```python
from build123d import *

# Parameters (mm, degrees)
SKETCH1_W           = 10
SKETCH1_H           = 10
BOSS_EXTRUDE1_DEPTH = 50
SKETCH3_R           = 4.25
BOSS_EXTRUDE2_DEPTH = 140
CHAMFER1_SIZE       = 1
SKETCH7_R           = 4
CUT_EXTRUDE3_DEPTH  = 4.5
SKETCH7_5_R         = 2.25
CUT_EXTRUDE4_DEPTH  = 20


with BuildPart() as part:
    # Sketch1 → Boss-Extrude1 (new body)
    with BuildSketch(Plane(origin=(0, 0, 0), x_dir=(0, 0, -1), z_dir=(1, 0, 0))):
        Rectangle(SKETCH1_W, SKETCH1_H)
    extrude(amount=BOSS_EXTRUDE1_DEPTH)

    # Sketch3 → Boss-Extrude2 (add)
    with BuildSketch(Plane(origin=(50, 0, 0), x_dir=(0, 0, -1), z_dir=(1, 0, 0))):
        Circle(SKETCH3_R)
    extrude(amount=BOSS_EXTRUDE2_DEPTH)

    # Chamfer1
    chamfer1_edges = [part.edges().sort_by_distance(p)[0] for p in [
        (190, 0, 4.25),
    ]]
    chamfer(chamfer1_edges, length=CHAMFER1_SIZE)

    # Sketch5 → Cut-Revolve1 (revolve, cut)
    with BuildSketch(Plane(origin=(0, 0, 0), x_dir=(-1, 0, 0), z_dir=(0, -0.7071067811865476, -0.7071067811865476))):
        Polygon((-50, 7.071067812), (-50, 6.571067812), (-49.5, 7.071067812), align=None)
    revolve(axis=Axis((-14.523088714, 0, 0), (1, 0, 0)), mode=Mode.SUBTRACT)

    # Sketch7 → Cut-Extrude3 (cut)
    with BuildSketch(Plane(origin=(0, 0, -5), x_dir=(-1, 0, 0), z_dir=(0, 0, -1))):
        with Locations(Location((-5, 0, 0), (0, 0, 90))):
            Circle(SKETCH7_R)
    extrude(amount=-CUT_EXTRUDE3_DEPTH, mode=Mode.SUBTRACT)

    # Sketch7_5 → Cut-Extrude4 (cut)
    with BuildSketch(Plane(origin=(0, 0, -5), x_dir=(-1, 0, 0), z_dir=(0, 0, -1))):
        with Locations(Location((-5, 0, 0), (0, 0, 90))):
            Circle(SKETCH7_5_R)
    extrude(amount=-CUT_EXTRUDE4_DEPTH, mode=Mode.SUBTRACT)


solid = part.part
```
CAD build for the part. Positions are in the model's coordinates, mm. A direction names the side the tool comes from. Coordinates: 2 decimals unless noted, no trailing zeros. Write each loop counter-clockwise with the first axis right and the second up, starting at its lowest first coordinate (ties: lowest second). Pieces come first, ordered by that corner, then holes. Notation, with made-up numbers: (68.5, -4.75) -> (111.5, -4.75) arc R19 ccw to (111.5, 5.25) -> close; hole circle Ø5 at (89.5, -20.5). An arc over 180 degrees is marked (long way). Use CSV: the item, a comma, the result in double quotes. Start each with the question number.
Item 1: Band-saw the part on C-C, the plane x = 96. Write the cut outline in (y, z), plus the area to 3 significant figures.
Item 2: Band-saw the part on B-B, the plane x = 5. Write the cut outline in (y, z), plus the area to 4 significant figures.
Item 3: Drop flat-ended pins along their axis: P1, Ø5, axis at x = 5, y = 0, coming from the +Z side; P2, Ø1, axis at x = 160.5, z = -2, coming from the +Y side; P3, Ø2.5, axis at x = 5, y = -1.5, coming from the -Z side; P4, Ø6, axis at x = 72, z = 4, coming from the -Y side. Give the stop position or say it passes through.
Item 4: Band-saw the part on A-A, the plane y = 0. Write the cut outline in (x, z), plus the area to 3 significant figures.
Item 5: Two-plate mould, pull along X, no slides. Class faces 1 (the flat face through (0, 0, 0)), 2 (the cylindrical face through (1.095, -0.867, -2.782)), 3 (the flat face through (25, 5, 0)), 4 (the flat face through (50, 4.5, 0.1)): +X half, -X half, draft (parallel to the pull), parting line (faces both ways), or undercut.
Item 6: Tool access for faces 5 (the flat face through (3, 2, -0.5)), 6 (the cylindrical face through (7.23, -0.29, 2.21)), 7 (the cylindrical face through (118.527, 3.584, -2.285)): list every direction of +Z, -Z, +X, -X, +Y, -Y with a clear straight run to the whole face (end or side of a thin tool).
Item 7: Wall check: probe 1 along X at (y, z) = (0, 1.25); probe 2 along X at (y, z) = (0, -3.1); probe 3 along Z at (x, y) = (137.5, 0.5). Give the ranges that are in metal, low to high.
Response values:
1,outline,"circle Ø8.5 at (0, 0)"
1,area,"56.7 mm2"
2,outline,"(-5, -5) -> (-4, -5) -> (-4, -0.5) -> (-2.25, -0.5) -> (-2.25, 5) -> (-5, 5) -> close; (2.25, -0.5) -> (4, -0.5) -> (4, -5) -> (5, -5) -> (5, 5) -> (2.25, 5) -> close"
2,area,"39.25 mm2"
3,P1,"stops at z = 5"
3,P2,"stops at y = 3.98"
3,P3,"stops at z = -0.5"
3,P4,"stops at y = -4.13"
4,outline,"(0, -5) -> (1, -5) -> (1, -0.5) -> (2.75, -0.5) -> (2.75, 5) -> (0, 5) -> close; (7.25, -0.5) -> (9, -0.5) -> (9, -5) -> (50, -5) -> (50, -4.25) -> (189, -4.25) -> (190, -3.25) -> (190, 3.25) -> (189, 4.25) -> (50, 4.25) -> (50, 5) -> (7.25, 5) -> close"
4,area,"1,630 mm2"
5,face 1,"-X half"
5,face 2,"undercut"
5,face 3,"draft"
5,face 4,"+X half"
6,face 5,"-Z"
6,face 6,"+Z, -Z"
6,face 7,"+X"
7,probe 1,"x = 0 to 2.75, 7.25 to 190"
7,probe 2,"x = 0 to 1, 9 to 190"
7,probe 3,"z = -4.22 to 4.22"
